from build123d import *

# Parameters (mm, degrees)
F0_W          = 200
F0_H          = 100
F1_DEPTH      = 15
F2_W          = 186.494716
F2_H          = 5.16998
F3_DEPTH      = 25.4
F3_DEPTH_BACK = 187.415063
F4_R          = 5


with BuildPart() as f1:
    # F0 (on Front) → F1 (new body)
    with BuildSketch(Plane.XZ):
        with Locations((0.974886, 12.01759)):
            Rectangle(F0_W, F0_H)
    extrude(amount=F1_DEPTH)

    # F2 (on face) → F3 (cut, two sides)
    with BuildSketch(Plane(origin=(0, 0, -37.98241), x_dir=(1, 0, 0), z_dir=(0, 0, -1))) as f3_sk:
        with Locations((0.691179, 7.258117)):
            Rectangle(F2_W, F2_H)
    extrude(amount=F3_DEPTH, mode=Mode.SUBTRACT)
    extrude(f3_sk.sketch, amount=-F3_DEPTH_BACK, mode=Mode.SUBTRACT)

    # F4
    f4_edges = [f1.edges().sort_by_distance(p)[0] for p in [
        (-99.025114, -7.5, 62.01759),
        (100.974886, -7.5, 62.01759),
        (100.974886, -7.5, -37.98241),
        (-99.025114, -7.5, -37.98241),
    ]]
    fillet(f4_edges, radius=F4_R)


solid = f1.part
Input: part model. Units: mm. Frame: model coordinates. A direction names the side the tool comes from. Coordinates: 2 decimals unless noted, no trailing zeros. Loops run counter-clockwise (first coordinate to the right, second up) from the corner with the lowest first, then second, coordinate; pieces in that order, holes last. Notation, with made-up numbers: (27.5, 2.25) - (50.5, 2.25) arc R10 cw to (50.5, 8.25) - close; hole circle Ø11 at (72, 73). An arc over 180 degrees is marked (long way). Answer in a Markdown table with one row per item. Add a question column.
Item 1: Section query A-A on x = 28. Return the cut outline in (y, z).
Item 2: Mould query, pull axis X, two halves, no side actions, for faces 1 (the flat face through (93.939, -7, 11)), 2 (the flat face through (-99.025, -7, 11)), 3 (the flat face through (100.975, -7, 11)). Classes: released by +X, released by -X, zero draft, split by the parting line, or undercut.
Item 3: Section query C-C on y = -8. Return the cut outline in (x, z).
Item 4: Access query for faces 4 (the cylindrical face through (-97.6, -7.6, -36.48)), 5 (the flat face through (-92.556, -7, 11)). Directions: +Z, -Z, +X, -X, +Y, -Y. A direction counts if a zero-diameter tool reaches every point of the face in a straight line with its end or side. Return the directions, or none.
Item 5: Section query B-B on z = 51. Return the cut outline in (x, y), then the cut area to 3 significant figures.
Item 6: Line query: line 1 along Y through (x, z) = (-84, 10); line 2 along X through (y, z) = (-6, -16.5). Output: solid intervals per line, ascending. Write a range as [from, to].
Recorded:
| question | item | result |
|---|---|---|
| 1 | outline | (-15, -37.98) - (-9.84, -37.98) - (-9.84, 62.02) - (-15, 62.02) - close; (-4.67, -37.98) - (0, -37.98) - (0, 62.02) - (-4.67, 62.02) - close |
| 2 | face 1 | undercut |
| 2 | face 2 | released by -X |
| 2 | face 3 | released by +X |
| 3 | outline | (-99.03, -32.98) arc R5 ccw to (-94.03, -37.98) - (-92.56, -37.98) - (-92.56, 62.02) - (-94.03, 62.02) arc R5 ccw to (-99.03, 57.02) - close; (93.94, -37.98) - (95.97, -37.98) arc R5 ccw to (100.97, -32.98) - (100.97, 57.02) arc R5 ccw to (95.97, 62.02) - (93.94, 62.02) - close |
| 4 | face 4 | -Z, -X, +Y, -Y |
| 4 | face 5 | +Z, -Z |
| 5 | outline | (-99.03, -15) - (100.97, -15) - (100.97, 0) - (-99.03, 0) - close; hole (-92.56, -9.84) - (93.94, -9.84) - (93.94, -4.67) - (-92.56, -4.67) - close |
| 5 | area | 2,040 mm^2 |
| 6 | line 1 | [-15, -9.84], [-4.67, 0] |
| 6 | line 2 | [-99.03, -92.56], [93.94, 100.97] |
